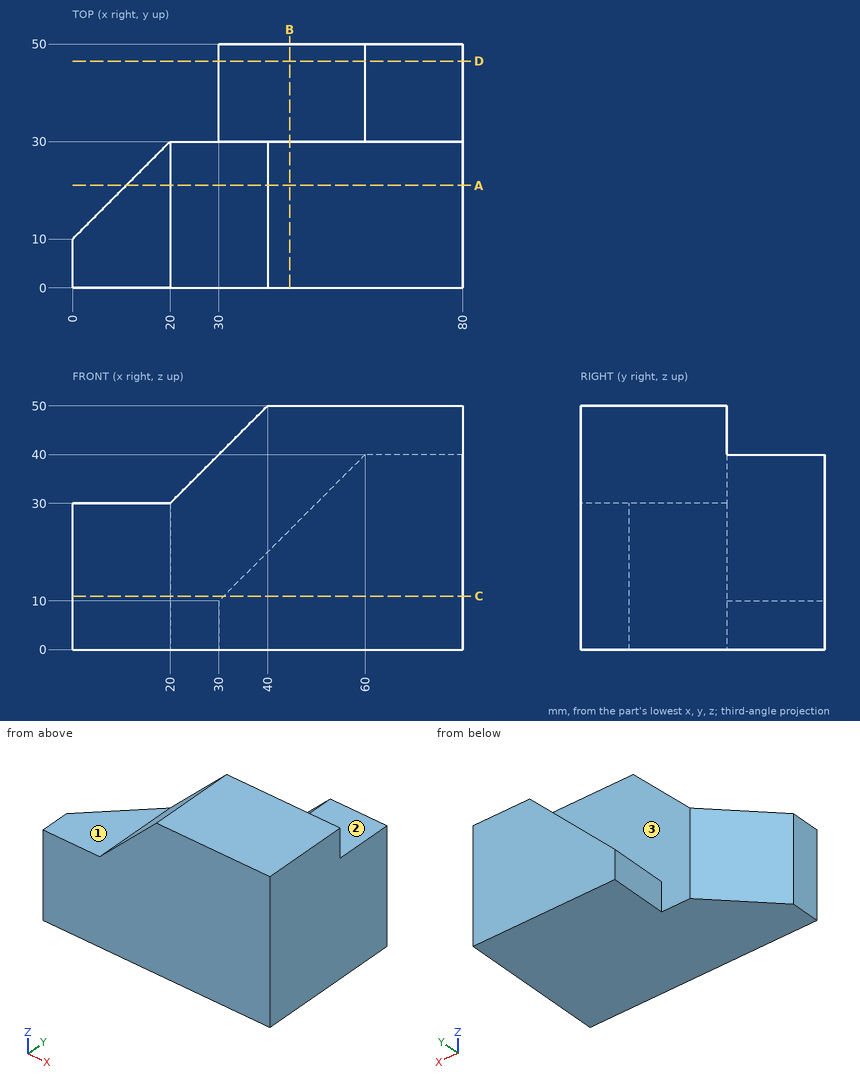
Can you work these out from the drawing? Everything is in mm from the part's minimum corner. A direction names the side the tool comes from. Round coordinates to 2 decimals unless told otherwise and drop trailing zeros. Order: outer loops, then holes, each group sorted by start corner. A loop starts at its lowest first (then second) coordinate and runs counter-clockwise, first axis right, second up. Notation, with made-up numbers: (57, 27.25) -> (77, 27.25) arc R15 cw to (77, 45.25) -> close; hole circle Ø6 at (45, 60). An arc over 180 degrees is marked (long way). Use CSV: the item, a comma, the result in double quotes.
1. I want a section at A-A on y = 21. List the corners of the cut face in (x, z) for me, and give its area (3 significant figures).
Recorded:
outline,"(11, 0) -> (80, 0) -> (80, 50) -> (40, 50) -> (20, 30) -> (11, 30) -> close"
area,"3,070 mm2"
2. I need wall thicknesses on line 1 along Y through (x, z) = (73, 45); line 2 along X through (y, z) = (35, 5). Which ranges of each line are inside material? Lowest first, please.
Recorded:
line 1,"y = 0 to 30"
line 2,"x = 30 to 80"
3. I'm going to push flat-ended pins straight in: P1, Ø3, axis at y = 44, z = 7, coming from the -X side; P2, Ø10, axis at x = 11.5, y = 17.5, coming from the +Z side; P3, Ø12, axis at y = 32.5, z = 27.5, coming from the -X side. Where does each tip first touch, or does it pass through?
Recorded:
P1,"stops at x = 30"
P2,"stops at z = 30"
P3,"stops at x = 16.5"
4. Which directions (+Z, -Z, +X, -X, +Y, -Y) give clear straight access to the entire face, cutting with the end or side of a thin tool? Please do the marked faces 1, 2 and 3.
Recorded:
face 1,"+Z, -X, +Y, -Y"
face 2,"+Z, +X, -X, +Y"
face 3,"+Z, -X, +Y"
5. I want a section at C-C on z = 11. List the corners of the cut face in (x, y) for me, and give its area (3 significant figures).
Recorded:
outline,"(0, 0) -> (80, 0) -> (80, 50) -> (31, 50) -> (31, 30) -> (20, 30) -> (0, 10) -> close"
area,"3,180 mm2"
6. I want a section at D-D on y = 46.5. List the corners of the cut face in (x, z) for me.
Recorded:
outline,"(30, 0) -> (80, 0) -> (80, 40) -> (60, 40) -> (30, 10) -> close"
7. I want a section at B-B on x = 44.5. List the corners of the cut face in (y, z) for me, and give its area (3 significant figures).
Recorded:
outline,"(0, 0) -> (50, 0) -> (50, 24.5) -> (30, 24.5) -> (30, 50) -> (0, 50) -> close"
area,"1,990 mm2"
